Part print with two shaded views. Sizes in mm from the minimum x, y, z corner. Coordinates: 2 decimals unless noted, no trailing zeros. Write each loop counter-clockwise with the first axis right and the second up, starting at its lowest first coordinate (ties: lowest second). Pieces come first, ordered by that corner, then holes.
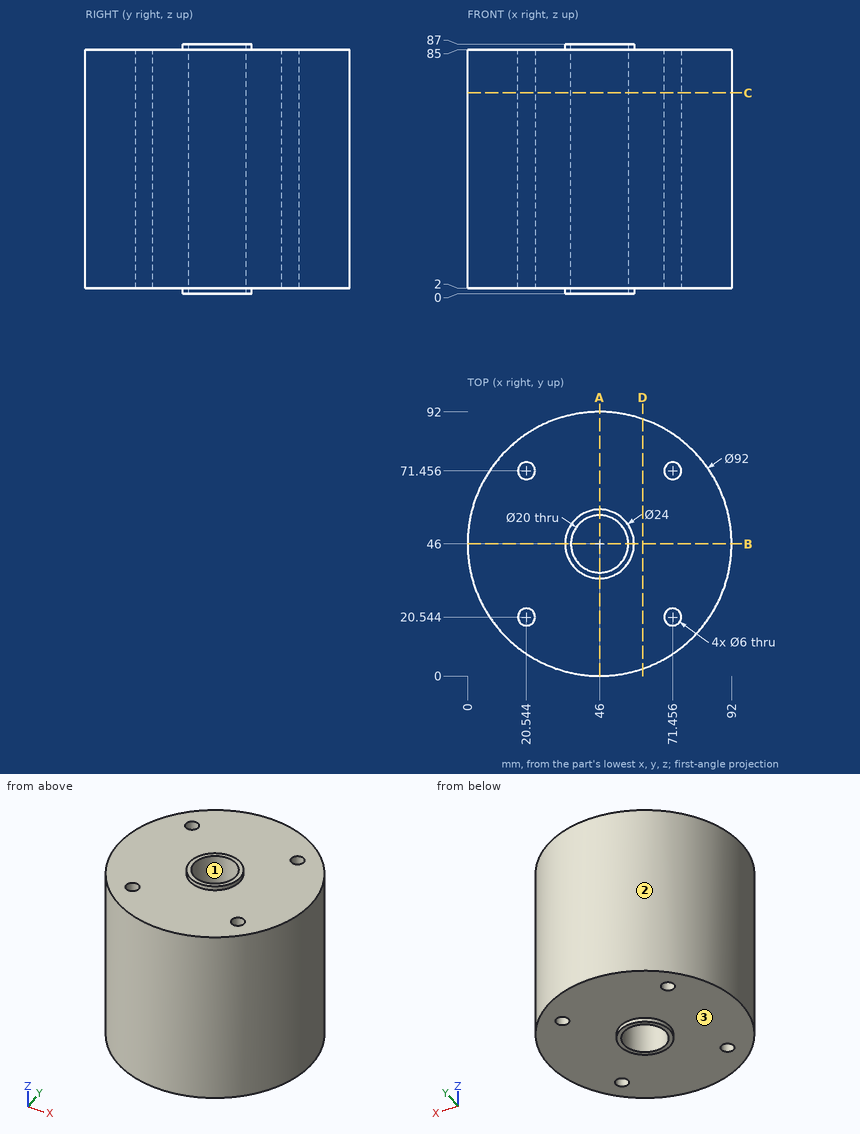
(1) Slice it at D-D, the plane x = 61. List the corners of the cut face in (y, z), and give its area (3 significant figures).
(2) Slice it at A-A, the plane x = 46. List the corners of the cut face in (y, z), and give its area (3 significant figures).
(3) Probe L1, parallel to Y at x = 46, z = 38.5; L2, parallel to X at y = 72, z = 64.5 (1 decimal); L3, parallel to X at y = 74, z = 38 (1 decimal). List the from-to ranges inside material, lowest first.
(4) Two-plate mould, pull along X, no slides. Class the marked faces 1, 2 and 3: pulls with the +X half, pulls with the -X half, needs draft (parallel to the pull), parting line crosses it, or undercut.
(5) Slice it at C-C, the plane z = 70. List the corners of the cut face in (x, y), and give its area (3 significant figures).
(6) Flat gauge pins, fed straight in: P1, Ø7, axis at x = 71.46, y = 20.54, coming from the -Z side; P2, Ø5, axis at x = 30.5, z = 72, coming from the +Y side (3 decimals); P3, Ø6, axis at y = 73.5, z = 56, coming from the +X side. Where does each tip first touch, or does it go through?
Results:
1. outline: (2.51, 2) - (89.49, 2) - (89.49, 85) - (2.51, 85) - close
1. area: 7,220 mm2
2. outline: (0, 2) - (34, 2) - (34, 0) - (36, 0) - (36, 87) - (34, 87) - (34, 85) - (0, 85) - close; (56, 0) - (58, 0) - (58, 2) - (92, 2) - (92, 85) - (58, 85) - (58, 87) - (56, 87) - close
2. area: 5,990 mm2
3. L1: y = 0 to 36, 56 to 92
3. L2: x = 8.1 to 17.6, 23.5 to 68.5, 74.4 to 83.9
3. L3: x = 9.5 to 19, 22.1 to 69.9, 73 to 82.5
4. face 1: undercut
4. face 2: parting line crosses it
4. face 3: needs draft
5. outline: circle Ø92 at (46, 46); hole circle Ø6 at (20.54, 20.54); hole circle Ø6 at (20.54, 71.46); hole circle Ø20 at (46, 46); hole circle Ø6 at (71.46, 20.54); hole circle Ø6 at (71.46, 71.46)
5. area: 6,220 mm2
6. P1: stops at z = 2
6. P2: stops at y = 90.125
6. P3: stops at x = 84.93
